Geometry check sheet. Reference: the model listing, model coordinates, mm. A direction names the side the tool comes from. Give positions to 0.01 mm unless a question says otherwise; leave off trailing zeros. Loops run counter-clockwise (first coordinate to the right, second up) from the corner with the lowest first, then second, coordinate; pieces in that order, holes last. Notation, with made-up numbers: (-36, 74) -> (-27, 74) arc R19 ccw to (-27, 99) -> close; hole circle Ø3 at (14, -39). An arc over 180 degrees is marked (long way). One line per question, with ' | ' between items.
from build123d import *

# Parameters (mm, degrees)
F1_DEPTH       = 35
F3_DEPTH       = 10
F4_D           = 3.3
F4_DEPTH       = 13.5
F4_CSINK_D     = 6.72
F4_CSINK_ANGLE = 90
F4_TIP         = 0.9914200214


with BuildPart() as f1:
    # F0 (on Front) → F1 (new body)
    with BuildSketch(Plane.XZ):
        with BuildLine():
            Line((-36.7157287525, 0), (0, 0))
            Line((0, 0), (0, 10))
            Line((0, 10), (-35, 10))
            ThreePointArc((-35, 10), (-35.4320432104, 4.9269406382), (-36.7157287525, 0))
        make_face()
        with BuildLine():
            Line((-47.5, 0), (-36.7157287525, 0))
            ThreePointArc((-36.7157287525, 0), (-35.4320432104, 4.9269406382), (-35, 10))
            Line((-35, 10), (-47.5, 10))
            Line((-47.5, 10), (-47.5, 0))
        make_face()
        with BuildLine():
            ThreePointArc((-35, 10), (-43.7867965644, 31.2132034356), (-65, 40))
            Line((-65, 40), (-65, 27.5))
            ThreePointArc((-65, 27.5), (-52.6256313292, 22.3743686708), (-47.5, 10))
            Line((-47.5, 10), (-35, 10))
        make_face()
    extrude(amount=F1_DEPTH)

    # F2 (on Right) → F3 (join)
    with BuildSketch(Plane.YZ):
        Polygon((-35, 0), (0, 0), (0, 35), (-12.5, 35), (-12.5, 25), (-22.5, 25), (-22.5, 35), (-35, 35), align=None)
    extrude(amount=-F3_DEPTH)

    # F4
    with Locations(Plane.YZ):
        with Locations((-29, 29.7529604286), (-6, 29.7529604286)):
            CounterSinkHole(F4_D / 2, F4_CSINK_D / 2, depth=F4_DEPTH, counter_sink_angle=F4_CSINK_ANGLE)
            with Locations((0, 0, -(F4_DEPTH + F4_TIP / 2))):  # 118° drill point
                Cone(0, F4_D / 2, F4_TIP, mode=Mode.SUBTRACT)


solid = f1.part
Item 1: Sectioned sample at D-D (y = -17). Record the cut outline in (x, z), plus the area to 3 significant figures.
Result:
outline: (-65, 27.5) arc R17.5 cw to (-47.5, 10) -> (-47.5, 0) -> (0, 0) -> (0, 25) -> (-10, 25) -> (-10, 10) -> (-35, 10) arc R30 ccw to (-65, 40) -> close | area: 1,090 mm2
Item 2: Set-up check for faces 1 (the face through (-5, -6, 35)), 2 (the face through (-5.913, -27.784, 30.868)), 3 (the face through (-47.5, -17, 5)), 4 (the face through (-5, -22.5, 30)), 5 (the face through (-22, -17, 10)): record each of +Z, -Z, +X, -X, +Y, -Y from which the full face is reachable in a straight line by a thin tool's end or side.
Result:
face 1: +Z, +X, +Y, -Y | face 2: +X | face 3: -Z, -X, +Y, -Y | face 4: +Z, +X | face 5: +Z, +Y, -Y
Item 3: Release check for a two-part mould opening along Y. For faces 6 (the face through (-65, -17, 34)), 7 (the face through (-40, 0, 16)), 8 (the face through (-5, -17, 25)) record: pulls with the +Y half, pulls with the -Y half, needs draft (parallel to the pull), parting line crosses it, or undercut.
Result:
face 6: needs draft | face 7: pulls with the +Y half | face 8: undercut
Item 4: Sectioned sample at C-C (x = -9). Record the cut outline in (y, z).
Result:
outline: (-35, 0) -> (0, 0) -> (0, 35) -> (-12.5, 35) -> (-12.5, 25) -> (-22.5, 25) -> (-22.5, 35) -> (-35, 35) -> close; hole circle Ø3.3 at (-29, 29.75); hole circle Ø3.3 at (-6, 29.75)
Item 5: Scan lines: probe 1 along Z at (x, y) = (-5, -29); probe 2 along X at (y, z) = (-25.5, 3); probe 3 along X at (y, z) = (-30.5, 32). Record each from-to range of solid material in increasing order.
Result:
probe 1: 0 to 28.1, 31.4 to 35 | probe 2: -47.5 to 0 | probe 3: -65 to -44.6, -10 to -0.66
Item 6: Depth check by flat-ended pin: pin 1 Ø8 at (x, y) = (-2.5, -7.5) entering from +Z; pin 2 Ø7.5 at (y, z) = (-12.5, 21.5) entering from -X; pin 3 Ø5.5 at (y, z) = (-6, 29.75) entering from +X. Enter the tip coordinate at first touch or a pass-through.
Result:
pin 1: z = 35 | pin 2: x = -56.42 | pin 3: x = -0.61
Item 7: Sectioned sample at A-A (y = -29). Record the cut outline in (x, z), plus the area to 3 significant figures.
Result:
outline: (-65, 27.5) arc R17.5 cw to (-47.5, 10) -> (-47.5, 0) -> (0, 0) -> (0, 26.39) -> (-1.71, 28.1) -> (-10, 28.1) -> (-10, 10) -> (-35, 10) arc R30 ccw to (-65, 40) -> close; (-10, 31.4) -> (-1.71, 31.4) -> (0, 33.11) -> (0, 35) -> (-10, 35) -> close | area: 1,160 mm2
Item 8: Sectioned sample at B-B (z = 15). Record the cut outline in (x, y), plus the area to 3 significant figures.
Result:
outline: (-48.23, -35) -> (-35.42, -35) -> (-35.42, 0) -> (-48.23, 0) -> close; (-10, -35) -> (0, -35) -> (0, 0) -> (-10, 0) -> close | area: 798 mm2
